Check sheet for the modelled part. Datum: model origin and axes. Units: mm. Face numbers are marked on the shaded views. A direction names the side the tool comes from. Give positions to 0.01 mm unless a question says otherwise; leave off trailing zeros. Order: outer loops, then holes, each group sorted by start corner. A loop starts at its lowest first (then second) coordinate and runs counter-clockwise, first axis right, second up. Notation, with made-up numbers: (40.25, -6.75) -> (53.25, -6.75) arc R18 ccw to (53.25, 7.25) -> close; hole circle Ø7 at (9.25, 7.25). An arc over 180 degrees is marked (long way). One line per question, with ' | ' between items.
Autodesk Fusion 360 part; units mm, degrees
sketch "Sketch1" plane through (0, 0, 0) normal (0, 1, 0) x (1, 0, 0)
  line L0 (-52.5, 33.75) -> (52.5, 33.75)
  line L1 (52.5, 33.75) -> (52.5, -33.75)
  line L2 (52.5, -33.75) -> (-52.5, -33.75)
  line L3 (-52.5, -33.75) -> (-52.5, 33.75)
  line L4 (-52.5, 33.75) -> (52.5, -33.75) construction
  dimension "d1" = 105
  dimension "d2" = 67.5
extrude "Extrude1" add sketch "Sketch1" along normal blind 3
sketch "Sketch2" plane through (0, 3, 0) normal (0, 1, 0) x (-1, 0, 0)
  line L0 (52.5, 33.75) -> (-52.5, 33.75)
  line L1 (-52.5, 33.75) -> (-52.5, -33.75)
  line L2 (-52.5, -33.75) -> (52.5, -33.75)
  line L3 (52.5, -33.75) -> (52.5, 33.75)
  line L4 (50.5, 31.75) -> (-50.5, 31.75)
  line L5 (-50.5, 31.75) -> (-50.5, -31.75)
  line L6 (-50.5, -31.75) -> (50.5, -31.75)
  line L7 (50.5, -31.75) -> (50.5, 31.75)
  dimension "d5" = -2
extrude "Extrude2" add sketch "Sketch2" along normal blind 20
sketch "Sketch3" plane through (0, 0, -33.75) normal (0, 0, -1) x (-1, 0, 0)
  line L0 (-52.5, 0) -> (52.5, 0)
  line L1 (52.5, 0) -> (52.5, 23)
  line L2 (52.5, 23) -> (-52.5, 23)
  line L3 (-52.5, 23) -> (-52.5, 0)
  line L4 (-40.5, 7.5) -> (-22.25, 7.5)
  line L5 (-22.25, 7.5) -> (-22.25, 3)
  line L6 (-22.25, 3) -> (-40.5, 3)
  line L7 (-40.5, 3) -> (-40.5, 7.5)
  dimension "d21" = 18.25
  dimension "d22" = 4.5
  dimension "d23" = 3
  dimension "d24" = 40.5
extrude "Extrude3" cut sketch "Sketch3" against normal blind 3 contours L4 L5 L6 L7
sketch "Sketch4" plane through (0, 3, 0) normal (0, 1, 0) x (-1, 0, 0)
  line L0 (-22.25, -31.75) -> (50.5, -31.75)
  line L1 (50.5, -31.75) -> (50.5, 31.75)
  line L2 (50.5, 31.75) -> (-50.5, 31.75)
  line L3 (-50.5, 31.75) -> (-50.5, -31.75)
  line L4 (-50.5, -31.75) -> (-40.5, -31.75)
  line L5 (-40.5, -31.75) -> (-40.5, -33.75)
  line L6 (-40.5, -33.75) -> (-22.25, -33.75)
  line L7 (-22.25, -33.75) -> (-22.25, -31.75)
  line L8 (46.5, -27.5) -> (-46.5, -27.5) construction
  line L9 (-46.5, -27.5) -> (-46.5, 27.5) construction
  line L10 (-46.5, 27.5) -> (46.5, 27.5) construction
  line L11 (46.5, 27.5) -> (46.5, -27.5) construction
  line L12 (46.5, -27.5) -> (-46.5, 27.5) construction
  circle A0 centre (46.5, -27.5) radius 1.5
  line L13 (50.5, -23.5) -> (42.5, -23.5)
  line L14 (42.5, -23.5) -> (42.5, -31.75)
  line L15 (50.5, 0) -> (-50.5, 0) construction
  line L16 (50.5, 23.5) -> (42.5, 23.5)
  line L17 (42.5, 23.5) -> (42.5, 31.75)
  circle A1 centre (46.5, 27.5) radius 1.5
  line L18 (0, -27.5) -> (0, 27.5) construction
  line L19 (-42.5, -23.5) -> (-42.5, -31.75)
  line L20 (-50.5, -23.5) -> (-42.5, -23.5)
  circle A2 centre (-46.5, -27.5) radius 1.5
  circle A3 centre (-46.5, 27.5) radius 1.5
  line L21 (-50.5, 23.5) -> (-42.5, 23.5)
  line L22 (-42.5, 23.5) -> (-42.5, 31.75)
  dimension "d33" = 93
  dimension "d34" = 55
  dimension "d35" = 3
  dimension "d36" = 4
  dimension "d37" = 4
extrude "Extrude4" add sketch "Sketch4" along normal blind 11 contours L0 L1 L13 L14 | L1 L2 L16 L17 | L3 L4 L19 L20 | L2 L3 L21 L22
fillet "Fillet1" radius 3 4 edges at (-50.5, 18.5, -31.75) (50.5, 18.5, -31.75) (50.5, 18.5, 31.75) (-50.5, 18.5, 31.75)
fillet "Fillet2" radius 5 4 edges at (-52.5, 11.5, 33.75) (52.5, 11.5, 33.75) (52.5, 11.5, -33.75) (-52.5, 11.5, -33.75)
sketch "Sketch5" plane through (0, 0, 33.75) normal (0, 0, 1) x (1, 0, 0)
  line L0 (47.5, 0) -> (47.5, 23)
  line L1 (47.5, 23) -> (-47.5, 23)
  line L2 (-47.5, 23) -> (-47.5, 0)
  line L3 (-47.5, 0) -> (47.5, 0)
  circle A0 centre (0, 7) radius 3
  line L4 (0, 7) -> (0, 0) construction
  dimension "d58" = 6
  dimension "d59" = 7
extrude "Extrude5" cut sketch "Sketch5" against normal blind 3 contours A0
sketch "Sketch6" plane through (0, 0, 33.75) normal (0, 0, 1) x (1, 0, 0)
  circle A0 centre (0, 7) radius 3
  line L0 (47.5, 0) -> (47.5, 23)
  line L1 (47.5, 23) -> (-47.5, 23)
  line L2 (-47.5, 23) -> (-47.5, 0)
  line L3 (-47.5, 0) -> (47.5, 0)
  line L4 (24, 10.5) -> (38.5, 10.5)
  line L5 (38.5, 10.5) -> (38.5, 3)
  line L6 (38.5, 3) -> (24, 3)
  line L7 (24, 3) -> (24, 10.5)
  dimension "d62" = 3
  dimension "d63" = 24
  dimension "d64" = 14.5
  dimension "d65" = 7.5
extrude "Extrude6" cut sketch "Sketch6" against normal blind 2 contours L4 L5 L6 L7
sketch "Sketch8" plane through (0, 3, 0) normal (0, 1, 0) x (-1, 0, 0)
  line L0 (-50.5, -23.5) -> (-42.5, -23.5)
  line L1 (-42.5, -23.5) -> (-42.5, -31.75)
  line L2 (-42.5, -31.75) -> (-40.5, -31.75)
  line L3 (-40.5, -31.75) -> (-40.5, -33.75)
  line L4 (-40.5, -33.75) -> (-22.25, -33.75)
  line L5 (-22.25, -33.75) -> (-22.25, -31.75)
  line L6 (-22.25, -31.75) -> (42.5, -31.75)
  line L7 (42.5, -31.75) -> (42.5, -23.5)
  line L8 (42.5, -23.5) -> (50.5, -23.5)
  line L9 (50.5, -23.5) -> (50.5, 23.5)
  line L10 (50.5, 23.5) -> (42.5, 23.5)
  line L11 (42.5, 23.5) -> (42.5, 31.75)
  line L12 (42.5, 31.75) -> (-24, 31.75)
  line L13 (-24, 31.75) -> (-24, 33.75)
  line L14 (-24, 33.75) -> (-38.5, 33.75)
  line L15 (-38.5, 33.75) -> (-38.5, 31.75)
  line L16 (-38.5, 31.75) -> (-42.5, 31.75)
  line L17 (-42.5, 31.75) -> (-42.5, 23.5)
  line L18 (-42.5, 23.5) -> (-50.5, 23.5)
  line L19 (-50.5, 23.5) -> (-50.5, -23.5)
  circle A0 centre (0, 0) radius 3
  dimension "d73" = 6
extrude "Extrude8" cut sketch "Sketch8" against normal blind 6 contours A0
chamfer "Chamfer1" distance 2 angle 45 1 edges at (2.797, 3, 1.0848)
sketch "Sketch9" plane through (-52.5, 0, 0) normal (-1, 0, 0) x (0, 0, 1)
  line L0 (-28.75, 23) -> (-28.75, 0)
  line L1 (-28.75, 0) -> (28.75, 0)
  line L2 (28.75, 0) -> (28.75, 23)
  line L3 (28.75, 23) -> (-28.75, 23)
  circle A0 centre (0, 8) radius 3.5
  line L4 (0, 8) -> (0, 0) construction
  dimension "d77" = 7
  dimension "d78" = 8
extrude "Extrude9" cut sketch "Sketch9" against normal blind 2 contours A0
fillet "Fillet3" radius 3.5 10 edges at (-42.5, 8.5, -23.5) (-50.5, 8.5, -23.5) (-42.5, 8.5, -31.75) (42.5, 8.5, -23.5) (50.5, 8.5, -23.5) (50.5, 8.5, 23.5) (42.5, 8.5, 23.5) (-42.5, 8.5, 31.75) (-42.5, 8.5, 23.5) (-50.5, 8.5, 23.5)
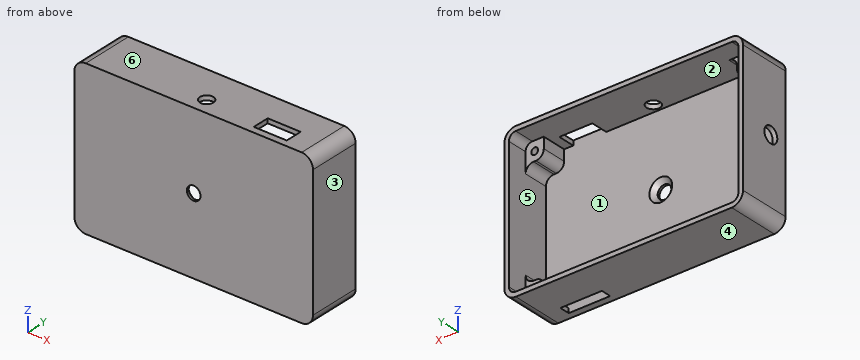
Q1. Section check A-A (y = 19.5). Enter the section's corners in (x, z).
Result sheet:
outline: (-52.5, -28.75) arc R5 ccw to (-47.5, -33.75) -> (47.5, -33.75) arc R5 ccw to (52.5, -28.75) -> (52.5, 28.75) arc R5 ccw to (47.5, 33.75) -> (-47.5, 33.75) arc R5 ccw to (-52.5, 28.75) -> close; hole (-50.5, -28.75) arc R3 ccw to (-47.5, -31.75) -> (47.5, -31.75) arc R3 ccw to (50.5, -28.75) -> (50.5, 28.75) arc R3 ccw to (47.5, 31.75) -> (-47.5, 31.75) arc R3 ccw to (-50.5, 28.75) -> close
Q2. Section check C-C (z = 14). Enter the section's corners in (x, y), and give its area (3 significant figures).
Result sheet:
outline: (-52.5, 0) -> (52.5, 0) -> (52.5, 23) -> (50.5, 23) -> (50.5, 3) -> (-50.5, 3) -> (-50.5, 23) -> (-52.5, 23) -> close | area: 395 mm2
Q3. Depth check by flat-ended pin: pin 1 Ø1.8 at (x, z) = (-46.5, -27.5) entering from -Y; pin 2 Ø1.6 at (y, z) = (6, -32.5) entering from -X; pin 3 Ø6 at (x, z) = (-44, -24.5) entering from +Y; pin 4 Ø2 at (y, z) = (7, 33) entering from +X. Enter the tip coordinate at first touch or a pass-through.
Result sheet:
pin 1: stops at y = 0 | pin 2: stops at x = -51.54 | pin 3: stops at y = 14 | pin 4: stops at x = 51.3
Q4. Section check B-B (x = 0). Enter the section's corners in (y, z).
Result sheet:
outline: (0, -33.75) -> (23, -33.75) -> (23, -31.75) -> (3, -31.75) -> (3, -5) -> (1, -3) -> (0, -3) -> close; (0, 3) -> (1, 3) -> (3, 5) -> (3, 31.75) -> (4, 31.75) -> (4, 33.75) -> (0, 33.75) -> close; (10, 31.75) -> (23, 31.75) -> (23, 33.75) -> (10, 33.75) -> close
Q5. Mould release check, pull along Z, two halves, no side actions. Record for the marked faces 1, 2, 3 and 4: pulls with the +Z half, pulls with the -Z half, needs draft (parallel to the pull), parting line crosses it, or undercut.
Result sheet:
face 1: undercut | face 2: undercut | face 3: needs draft | face 4: pulls with the -Z half
Q6. Thickness scan on line 1 (Z direction, x = -46.5, y = 9); line 2 (Y direction, x = 0, z = 32.5); line 3 (Z direction, x = 0, y = 0.3). Record the ranges inside material, lowest first.
Result sheet:
line 1: z = -33.75 to -29, -26 to -23.5, 23.5 to 26, 29 to 33.75 | line 2: y = 0 to 4, 10 to 23 | line 3: z = -33.75 to -3, 3 to 33.75
Q7. Access from +Z, -Z, +X, -X, +Y, -Y to the whole of each face (thin tool, end or side, straight path). Record for the marked faces 5 and 6.
Result sheet:
face 5: +Y | face 6: +Z, +X, -X, +Y, -Y
Q8. Section check D-D (x = -30). Enter the section's corners in (y, z), and give its area (4 significant figures).
Result sheet:
outline: (0, -33.75) -> (23, -33.75) -> (23, -31.75) -> (3, -31.75) -> (3, 31.75) -> (23, 31.75) -> (23, 33.75) -> (0, 33.75) -> close | area: 282.5 mm2
